from build123d import *

# Parameters (mm, degrees)
ESBO_O3_R                = 5
RESSALTO_EXTRUS_O1_DEPTH = 15


with BuildPart() as part:
    # Esboço1 → Revolução1 (revolve)
    with BuildSketch(Plane.XY):
        Polygon((0, 200), (9, 200), (9, 0), (25, 0), (25, -8), (0, -8), (0, 0), align=None)
    revolve(axis=Axis((0, 0, 0), (0, 1, 0)))

    # Esboço3 → Ressalto-extrusão1 (add, symmetric)
    with BuildSketch(Plane.XY):
        with BuildLine():
            Line((-10, -8), (10, -8))
            Line((10, -8), (10, -38))
            ThreePointArc((10, -38), (0, -48), (-10, -38))
            Line((-10, -38), (-10, -8))
        make_face()
        with Locations((0, -38)):
            Circle(ESBO_O3_R, mode=Mode.SUBTRACT)
    extrude(amount=RESSALTO_EXTRUS_O1_DEPTH, both=True)


solid = part.part
For this review, take the finished solid that the model builds, in its own axes (mm). A direction names the side the tool comes from. Round coordinates to 2 decimals unless told otherwise and drop trailing zeros. Order: outer loops, then holes, each group sorted by start corner. A loop starts at its lowest first (then second) coordinate and runs counter-clockwise, first axis right, second up. Notation, with made-up numbers: M 88,3 L 141,3 A13 cw 141,28 Z; hole C 50.25,-8.5 d3. An arc over 180 degrees is marked long. Use a Markdown table: item, result. Add a question column.
Item 1: Insertion check: pin 1 (12 mm diameter, centred on x = 7, y = 135, fed in from -Z); pin 2 (10 mm diameter, centred on x = -2, y = -26.5, fed in from -Z); pin 3 (1.5 mm diameter, centred on x = -7, y = 73.5, fed in from -Z). Each pin has a flat end and moves straight along its axis. Give the tip position at first contact, or say it passes through.
Item 2: Add section A-A, the plane x = 0. Give the boundary of the cut face in (y, z), then the cut area to 3 significant figures.
Item 3: Mouldability with a two-part tool opening along X and no side actions: class faces 4 (the cylindrical face through (23.846, -4.056, -7.509)), 5 (the cylindrical face through (3, -34, 0)), 6 (the flat face through (10, -23, 0)), 7 (the flat face through (11, -8, 0)) as released by +X, released by -X, zero draft, split by the parting line, or undercut.
Item 4: Add section D-D, the plane y = 99. Give the boundary of the cut face in (x, z), then the cut area to 3 significant figures.
Item 5: Tool access review of faces 1 (the cylindrical face through (-1.172, 98.6, -8.923)), 2 (the flat face through (0, -28, 15)), 3 (the flat face through (-10, -23, 0)): name each direction out of +Z, -Z, +X, -X, +Y, -Y from which nothing blocks a thin tool from reaching the whole face with its end or side.
Item 6: To check wall thickness, follow line 1 along Y through (x, z) = (0, 5.75); line 2 along X through (y, z) = (-26, -12); line 3 along Y through (x, z) = (-21.5, -4). State the ranges of each line that lie inside material, in increasing order.
Item 7: Add section B-B, the plane z = 0. Give the boundary of the cut face in (x, y).
Item 8: Add section C-C, the plane y = -19. Give the boundary of the cut face in (x, z).
Geometry results:
| question | item | result |
|---|---|---|
| 1 | pin 1 | stops at z = -8.94 |
| 1 | pin 2 | stops at z = -15 |
| 1 | pin 3 | stops at z = -6.48 |
| 2 | outline | M -48,-15 L -43,-15 L -43,15 L -48,15 Z; M -33,-15 L -8,-15 L -8,-25 L 0,-25 L 0,-9 L 200,-9 L 200,9 L 0,9 L 0,25 L -8,25 L -8,15 L -33,15 Z |
| 2 | area | 4,900 mm² |
| 3 | face 4 | split by the parting line |
| 3 | face 5 | undercut |
| 3 | face 6 | released by +X |
| 3 | face 7 | zero draft |
| 4 | outline | C 0,0 d18 |
| 4 | area | 254 mm² |
| 5 | face 1 | +Y |
| 5 | face 2 | +Z, +X, -X, -Y |
| 5 | face 3 | +Z, -Z, -X, -Y |
| 6 | line 1 | y = -48 to -43, -33 to 200 |
| 6 | line 2 | x = -10 to 10 |
| 6 | line 3 | y = -8 to 0 |
| 7 | outline | M -25,-8 L -10,-8 L -10,-38 A10 ccw 10,-38 L 10,-8 L 25,-8 L 25,0 L 9,0 L 9,200 L -9,200 L -9,0 L -25,0 Z; hole C 0,-38 d10 |
| 8 | outline | M -10,-15 L 10,-15 L 10,15 L -10,15 Z |
